from build123d import *

# Parameters (mm, degrees)
CHAMFER1_SIZE = 0.8


with BuildPart() as part:
    # Sketch2 → Revolve1 (revolve)
    with BuildSketch(Plane(origin=(0, 0, 0), x_dir=(1, 0, 0), z_dir=(0, 1, 0))):
        Polygon((1.65, 18.8), (1.65, 0), (9.5, 0), (9.5, 2), (6, 2), (6, 3.5), (8.5, 3.5), (8.5, 4.4), (3.5, 4.4), (3.5, 5.9), (8.5, 5.9), (8.5, 6.8), (3.5, 6.8), (3.5, 8.3), (8.5, 8.3), (8.5, 9.2), (3.5, 9.2), (3.5, 10.7), (8.5, 10.7), (8.5, 11.6), (3.5, 11.6), (3.5, 13.1), (8.5, 13.1), (8.5, 14), (3.5, 14), (3.5, 15.5), (8.5, 15.5), (8.5, 16.4), (3.5, 16.4), (3.5, 17.9), (8.5, 17.9), (8.5, 18.8), align=None)
    revolve(axis=Axis((0, 0, 0), (0, 0, -1)))

    # Chamfer1
    chamfer1_edges = [part.edges().sort_by_distance(p)[0] for p in [
        (-1.65, 0, 0),
    ]]
    chamfer(chamfer1_edges, length=CHAMFER1_SIZE)

    # Sketch4 → Cut-Revolve1 (revolve, cut)
    with BuildSketch(Plane(origin=(0, 0, 0), x_dir=(1, 0, 0), z_dir=(0, 1, 0)), mode=Mode.PRIVATE) as cut_revolve1_sk:
        Polygon((0, 7.529612721), (1.65, 7.529612721), (2.1, 7.8), (2.1, 11.559655752), (2.5, 11.8), (2.5, 18.8), (0, 18.8), align=None)
    revolve(cut_revolve1_sk.sketch.rotate(Axis((0, 0, -18.8), (0, 0, 1)), 180), axis=Axis((0, 0, -18.8), (0, 0, 1)), mode=Mode.SUBTRACT)


solid = part.part
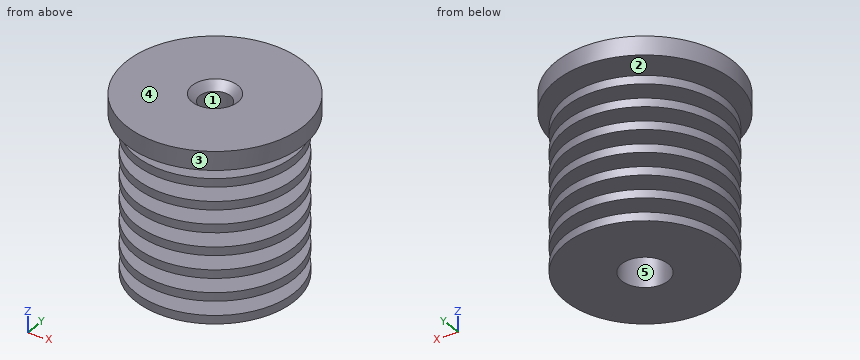
Verification items for the finished model (mm, model axes). Face numbers are marked on the shaded views. A direction names the side the tool comes from. Give positions to 0.01 mm unless a question says otherwise; leave off trailing zeros. Loops run counter-clockwise (first coordinate to the right, second up) from the corner with the lowest first, then second, coordinate; pieces in that order, holes last. Notation, with made-up numbers: (35.5, 33) - (64.5, 33) arc R29 ccw to (64.5, 62) - close; hole circle Ø9 at (-22, 39). An arc over 180 degrees is marked (long way). Write item = value, one per line. Start each with the question number.
Q1. Tool access check on the marked faces 4 and 5. Record the directions out of +Z, -Z, +X, -X, +Y, -Y that give a thin tool (end or side, any length) a straight path to the whole face; none if there is none.
Q2. Depth check by flat-ended pin: P1, Ø1.5, axis at y = 5.5, z = -3.5, coming from the +X side; P2, Ø2.5, axis at x = 0, y = 0, coming from the -Z side; P3, Ø3, axis at y = 2.5, z = -2, coming from the -X side; P4, Ø10, axis at y = -5.5, z = -16, coming from the +X side. Enter the tip coordinate at first touch or a pass-through.
Q3. Cross-section at B-B, the plane x = 6.5. State how many separate pieces and enclosed holes the cut face has, and give its area (3 significant figures).
Q4. Thickness scan on line 1 (Y direction, x = 0, z = -14.5); line 2 (Y direction, x = 0, z = -2.5); line 3 (X direction, y = 0, z = -4). Record the ranges inside material, lowest first.
Q5. Mould release check, pull along X, two halves, no side actions. Record for the marked faces 1, 2 and 3: released by +X, released by -X, zero draft, split by the parting line, or undercut.
Q6. Cross-section at C-C, the plane z = -16. Enter the section's corners in (x, y), and give its area (3 significant figures).
Q7. Cross-section at A-A, the plane z = -10. Enter the section's corners in (x, y), and give its area (3 significant figures).
Answer key:
q1.face_4 = +Z, +X, -X, +Y, -Y
q1.face_5 = -Z
q2.P1 = 7.05
q2.P2 = through
q2.P3 = -9.45
q2.P4 = 8.49
q3.separate_pieces = 8
q3.enclosed_holes = 0
q3.area = 96.7 mm^2
q4.line_1 = -3.5 to -2.5, 2.5 to 3.5
q4.line_2 = -6 to -1.65, 1.65 to 6
q4.line_3 = -8.5 to -1.65, 1.65 to 8.5
q5.face_1 = undercut
q5.face_2 = zero draft
q5.face_3 = split by the parting line
q6.outline = circle Ø17 at (0, 0); hole circle Ø5 at (0, 0)
q6.area = 207 mm^2
q7.outline = circle Ø7 at (0, 0); hole circle Ø4.2 at (0, 0)
q7.area = 24.6 mm^2
